from build123d import *

# Parameters (mm, degrees)
SKETCH_1_W          = 80
SKETCH_1_H          = 20
SKETCH_1_R          = 1
EXTRUDE_1_DEPTH     = 1.6
CUT_EXTRUDE_1_DEPTH = 0.1
CUT_EXTRUDE_START   = -0.1
CUT_EXTRUDE_2_DEPTH = 0.1


with BuildPart() as part:
    # Эскиз1 → Бобышка-Вытянуть1 (new body)
    with BuildSketch(Plane.XY):
        Rectangle(SKETCH_1_W, SKETCH_1_H)
        with Locations((-37.5, 7.5)):
            Circle(SKETCH_1_R, mode=Mode.SUBTRACT)
        with Locations((-37.5, -7.5)):
            Circle(SKETCH_1_R, mode=Mode.SUBTRACT)
        with Locations((37.5, -7.5)):
            Circle(SKETCH_1_R, mode=Mode.SUBTRACT)
        with Locations((37.5, 7.5)):
            Circle(SKETCH_1_R, mode=Mode.SUBTRACT)
    extrude(amount=EXTRUDE_1_DEPTH)

    # Эскиз2 → Вырез-Вытянуть1 (cut)
    with BuildSketch(Plane.XY.offset(1.6)):
        with BuildLine():
            Line((-38, -2.625), (-35, -2.625))
            ThreePointArc((-35, -2.625), (-33.625, -4), (-35, -5.375))
            Line((-35, -5.375), (-38, -5.375))
            ThreePointArc((-38, -5.375), (-39.375, -4), (-38, -2.625))
        make_face()
        with BuildLine():
            Line((-38, 1.375), (-35, 1.375))
            ThreePointArc((-35, 1.375), (-33.625, 0), (-35, -1.375))
            Line((-35, -1.375), (-38, -1.375))
            ThreePointArc((-38, -1.375), (-39.375, 0), (-38, 1.375))
        make_face()
        with BuildLine():
            Line((-38, 5.375), (-35, 5.375))
            ThreePointArc((-35, 5.375), (-33.625, 4), (-35, 2.625))
            Line((-35, 2.625), (-38, 2.625))
            ThreePointArc((-38, 2.625), (-39.375, 4), (-38, 5.375))
        make_face()
        with BuildLine():
            Line((38, -2.625), (35, -2.625))
            ThreePointArc((35, -2.625), (33.625, -4), (35, -5.375))
            Line((35, -5.375), (38, -5.375))
            ThreePointArc((38, -5.375), (39.375, -4), (38, -2.625))
        make_face()
        with BuildLine():
            Line((38, 1.375), (35, 1.375))
            ThreePointArc((35, 1.375), (33.625, 0), (35, -1.375))
            Line((35, -1.375), (38, -1.375))
            ThreePointArc((38, -1.375), (39.375, 0), (38, 1.375))
        make_face()
        with BuildLine():
            Line((38, 5.375), (35, 5.375))
            ThreePointArc((35, 5.375), (33.625, 4), (35, 2.625))
            Line((35, 2.625), (38, 2.625))
            ThreePointArc((38, 2.625), (39.375, 4), (38, 5.375))
        make_face()
    extrude(amount=-CUT_EXTRUDE_1_DEPTH, mode=Mode.SUBTRACT)

    # Эскиз3 → Вырез-Вытянуть2 (cut)
    with BuildSketch(Plane(origin=(0, 0, 0), x_dir=(-1, 0, 0), z_dir=(0, 0, -1)).offset(CUT_EXTRUDE_START)):
        with BuildLine():
            Line((38, 1.375), (35, 1.375))
            ThreePointArc((35, 1.375), (33.625, 0), (35, -1.375))
            Line((35, -1.375), (38, -1.375))
            ThreePointArc((38, -1.375), (39.375, 0), (38, 1.375))
        make_face()
        with BuildLine():
            Line((38, -2.625), (35, -2.625))
            ThreePointArc((35, -2.625), (33.625, -4), (35, -5.375))
            Line((35, -5.375), (38, -5.375))
            ThreePointArc((38, -5.375), (39.375, -4), (38, -2.625))
        make_face()
        with BuildLine():
            Line((38, 5.375), (35, 5.375))
            ThreePointArc((35, 5.375), (33.625, 4), (35, 2.625))
            Line((35, 2.625), (38, 2.625))
            ThreePointArc((38, 2.625), (39.375, 4), (38, 5.375))
        make_face()
        with BuildLine():
            Line((-35, 1.375), (-38, 1.375))
            ThreePointArc((-38, 1.375), (-39.375, 0), (-38, -1.375))
            Line((-38, -1.375), (-35, -1.375))
            ThreePointArc((-35, -1.375), (-33.625, 0), (-35, 1.375))
        make_face()
        with BuildLine():
            Line((-35, -2.625), (-38, -2.625))
            ThreePointArc((-38, -2.625), (-39.375, -4), (-38, -5.375))
            Line((-38, -5.375), (-35, -5.375))
            ThreePointArc((-35, -5.375), (-33.625, -4), (-35, -2.625))
        make_face()
        with BuildLine():
            Line((-35, 5.375), (-38, 5.375))
            ThreePointArc((-38, 5.375), (-39.375, 4), (-38, 2.625))
            Line((-38, 2.625), (-35, 2.625))
            ThreePointArc((-35, 2.625), (-33.625, 4), (-35, 5.375))
        make_face()
    extrude(amount=CUT_EXTRUDE_2_DEPTH, mode=Mode.SUBTRACT)


solid = part.part
Verification items for the finished model (mm, model axes). A direction names the side the tool comes from. Coordinates: 2 decimals unless noted, no trailing zeros. Order: outer loops, then holes, each group sorted by start corner. A loop starts at its lowest first (then second) coordinate and runs counter-clockwise, first axis right, second up. Notation, with made-up numbers: M 83,67.5 L 128,67.5 A31 ccw 128,97.5 Z; hole C 22.5,83.25 d10. An arc over 180 degrees is marked long. Return JSON: item names as keys, results as strings.
1) Access from +Z, -Z, +X, -X, +Y, -Y to the whole of each face (thin tool, end or side, straight path). Record for faces 1 (the flat face through (36, -4, 1.5)), 2 (the cylindrical face through (-36.546, -7.2, 0.789)), 3 (the flat face through (-36, -4, 0.1)).
Answer list:
{"face 1": "+Z", "face 2": "+Z, -Z", "face 3": "-Z"}
2) Gauge pin test, flat ends, axial feed: pin 1 (3 mm diameter, centred on x = -36.5, y = 0, fed in from -Z); pin 2 (0.8 mm diameter, centred on x = 37.5, y = 4, fed in from -Z). Record the tip position at first contact, or that the pin passes through.
Answer list:
{"pin 1": "z = 0", "pin 2": "z = 0.1"}
3) Cross-section at A-A, the plane y = 7.5. Record the boundary of the cut face in (x, z).
Answer list:
{"outline": "M -40,0 L -38.5,0 L -38.5,1.6 L -40,1.6 Z; M -36.5,0 L 36.5,0 L 36.5,1.6 L -36.5,1.6 Z; M 38.5,0 L 40,0 L 40,1.6 L 38.5,1.6 Z"}
4) Release check for a two-part mould opening along X. For faces 4 (the flat face through (-1, -10, 1)), 5 (the flat face through (-40, 0, 1)), 6 (the flat face through (-36, 0, 0.1)) record: +X half, -X half, draft (parallel to the pull), parting line (faces both ways), or undercut.
Answer list:
{"face 4": "draft", "face 5": "-X half", "face 6": "undercut"}
5) Thickness scan on L1, parallel to Y at x = 37.5, z = 1.15; L2, parallel to X at y = 7.75, z = 1.25; L3, parallel to X at y = 8, z = 0.95. Record the ranges inside material, lowest first. Write a range as [from, to].
Answer list:
{"L1": "[-10, -8.5], [-6.5, 6.5], [8.5, 10]", "L2": "[-40, -38.47], [-36.53, 36.53], [38.47, 40]", "L3": "[-40, -38.37], [-36.63, 36.63], [38.37, 40]"}
6) Cross-section at B-B, the plane y = 4. Record the boundary of the cut face in (x, z) (3 decimals), and give its area (3 significant figures).
Answer list:
{"outline": "M -40,0 L -39.375,0 L -39.375,0.1 L -33.625,0.1 L -33.625,0 L 33.625,0 L 33.625,0.1 L 39.375,0.1 L 39.375,0 L 40,0 L 40,1.6 L 39.375,1.6 L 39.375,1.5 L 33.625,1.5 L 33.625,1.6 L -33.625,1.6 L -33.625,1.5 L -39.375,1.5 L -39.375,1.6 L -40,1.6 Z", "area": "126 mm2"}
